Verification items for the finished model (mm, model axes). A direction names the side the tool comes from. Give positions to 0.01 mm unless a question says otherwise; leave off trailing zeros. Order: outer loops, then holes, each group sorted by start corner. A loop starts at its lowest first (then second) coordinate and runs counter-clockwise, first axis right, second up. Notation, with made-up numbers: (81, 52) - (128, 52) arc R10 ccw to (128, 71) - close; hole circle Ø11 at (-31, 26.25). An arc over 180 degrees is marked (long way). Answer as a JSON object with one key per item and string values. Group by question number.
(1) Access from +Z, -Z, +X, -X, +Y, -Y to the whole of each face (thin tool, end or side, straight path). Record for faces 3 (the face through (-0.5, -1, 3)), 4 (the face through (0, -53, 0)), 5 (the face through (0, 24, 1)).
(2) Section check A-A (z = 3.55). Record the boundary of the cut face in (x, y), then the cut area to 3 significant figures.
(3) Mould release check, pull along Z, two halves, no side actions. Record for faces 1 (the face through (0, -26, 0)), 2 (the face through (0, -55.52, 1.7)): +Z half, -Z half, draft (parallel to the pull), parting line (faces both ways), or undercut.
(4) Thickness scan on line 1 (X direction, y = -23, z = 3.55); line 2 (Y direction, x = 2, z = 4.6); line 3 (Z direction, x = -0.1, y = -35.5). Record the ranges inside material, lowest first.
(5) Section check B-B (y = 21). Record the boundary of the cut face in (x, z), then the cut area to 3 significant figures.
(6) Depth check by flat-ended pin: pin 1 Ø1.1 at (x, y) = (0, 8) entering from +Z; pin 2 Ø0.6 at (x, y) = (0, 39.5) entering from -Z. Enter the tip coordinate at first touch or a pass-through.
```python
from build123d import *

# Parameters (mm, degrees)
F0_W     = 0.5
F0_H     = 110
F1_DEPTH = 2
F0_W_2   = 2
F2_DEPTH = 5
F3_R     = 0.5
F4_W     = 2
F4_H     = 1
F5_DEPTH = 28.67605


with BuildPart() as f1:
    # F0 (on Top) → F1 (new body)
    with BuildSketch(Plane.XY):
        with Locations((-0.25, -0.5195)):
            Rectangle(F0_W, F0_H)
        with Locations((0.25, -0.5195)):
            Rectangle(F0_W, F0_H)
    extrude(amount=F1_DEPTH)

    # F0 (on Top) → F2 (join)
    with BuildSketch(Plane.XY):
        with Locations((-1.5, -0.5195)):
            Rectangle(F0_W_2, F0_H)
        with Locations((1.5, -0.5195)):
            Rectangle(F0_W_2, F0_H)
    extrude(amount=F2_DEPTH)

    # F3
    f3_edges = [f1.edges().sort_by_distance(p)[0] for p in [
        (-2.5, -55.5195, 2.5),
        (-1.5, -55.5195, 5),
        (1.5, -55.5195, 5),
        (2.5, -55.5195, 2.5),
        (2.5, -0.5195, 5),
        (-2.5, -0.5195, 5),
        (-1.5, 54.4805, 5),
        (1.5, 54.4805, 5),
        (2.5, 54.4805, 2.5),
        (-2.5, 54.4805, 2.5),
    ]]
    fillet(f3_edges, radius=F3_R)

    # F4 (on face) → F5 (cut)
    with BuildSketch(Plane(origin=(-2.5, 0, 0), x_dir=(0, -1, 0), z_dir=(-1, 0, 0))):
        with Locations((-50.451858, 0.5)):
            Rectangle(F4_W, F4_H)
        with Locations((-45.151858, 0.5)):
            Rectangle(F4_W, F4_H)
        with Locations((-39.851858, 0.5)):
            Rectangle(F4_W, F4_H)
        with Locations((-34.551858, 0.5)):
            Rectangle(F4_W, F4_H)
        with Locations((-29.251858, 0.5)):
            Rectangle(F4_W, F4_H)
        with Locations((-23.951858, 0.5)):
            Rectangle(F4_W, F4_H)
        with Locations((-18.651858, 0.5)):
            Rectangle(F4_W, F4_H)
        with Locations((-13.351858, 0.5)):
            Rectangle(F4_W, F4_H)
        with Locations((-8.051858, 0.5)):
            Rectangle(F4_W, F4_H)
        with Locations((-2.751858, 0.5)):
            Rectangle(F4_W, F4_H)
        with Locations((2.548142, 0.5)):
            Rectangle(F4_W, F4_H)
        with Locations((7.848142, 0.5)):
            Rectangle(F4_W, F4_H)
        with Locations((13.148142, 0.5)):
            Rectangle(F4_W, F4_H)
        with Locations((18.448142, 0.5)):
            Rectangle(F4_W, F4_H)
        with Locations((23.748142, 0.5)):
            Rectangle(F4_W, F4_H)
        with Locations((29.048142, 0.5)):
            Rectangle(F4_W, F4_H)
        with Locations((34.348142, 0.5)):
            Rectangle(F4_W, F4_H)
        with Locations((39.648142, 0.5)):
            Rectangle(F4_W, F4_H)
        with Locations((44.948142, 0.5)):
            Rectangle(F4_W, F4_H)
        with Locations((50.248142, 0.5)):
            Rectangle(F4_W, F4_H)
    extrude(amount=-F5_DEPTH, mode=Mode.SUBTRACT)


solid = f1.part
```
Solutions:
{
 "1": {"face 3": "+Z, +Y, -Y", "face 4": "-Z, +X, -X, +Y, -Y", "face 5": "-Z, +X, -X"},
 "2": {"outline": "(-2.5, -55.02) arc R0.5 ccw to (-2, -55.52) - (-0.5, -55.52) - (-0.5, 54.48) - (-2, 54.48) arc R0.5 ccw to (-2.5, 53.98) - close; (0.5, -55.52) - (2, -55.52) arc R0.5 ccw to (2.5, -55.02) - (2.5, 53.98) arc R0.5 ccw to (2, 54.48) - (0.5, 54.48) - close", "area": "440 mm2"},
 "3": {"face 1": "-Z half", "face 2": "draft"},
 "4": {"line 1": "x = -2.5 to -0.5, 0.5 to 2.5", "line 2": "y = -55.51 to 54.47", "line 3": "z = 0 to 2"},
 "5": {"outline": "(-2.5, 0) - (2.5, 0) - (2.5, 4.5) arc R0.5 ccw to (2, 5) - (0.5, 5) - (0.5, 2) - (-0.5, 2) - (-0.5, 5) - (-2, 5) arc R0.5 ccw to (-2.5, 4.5) - close", "area": "21.9 mm2"},
 "6": {"pin 1": "stops at z = 5", "pin 2": "stops at z = 1"}
}
